Could you check a few things on this model? Use its own coordinates, in mm. A direction names the side the tool comes from. Coordinates: 2 decimals unless noted, no trailing zeros. Order: outer loops, then holes, each group sorted by start corner. A loop starts at its lowest first (then second) coordinate and runs counter-clockwise, first axis right, second up. Notation, with made-up numbers: (57.5, 33) - (101.5, 33) arc R33 ccw to (101.5, 67) - close; hole circle Ø6 at (33, 28.5). An arc over 180 degrees is marked (long way). One line per item, written item: value.
from build123d import *

# Parameters (mm, degrees)
F1_DEPTH = 500
F2_R     = 5
F3_DEPTH = 3.7
F4_R     = 5
F5_DEPTH = 41.001


with BuildPart() as f1:
    # F0 (on Top) → F1 (new body)
    with BuildSketch(Plane.XY):
        Polygon((0, 41), (0, 0), (41, 0), (41, 41), (31.4, 41), (31.4, 34), (34.8, 34), (34.8, 37.5), (37.3, 37.5), (37.3, 3.7), (3.7, 3.7), (3.7, 37.5), (6.2, 37.5), (6.2, 34), (9.6, 34), (9.6, 41), align=None)
    extrude(amount=F1_DEPTH)

    # F2 (on face) → F3 (cut, through all)
    with BuildSketch(Plane(origin=(0, 3.7, 0), x_dir=(-1, 0, 0), z_dir=(0, 1, 0))):
        with Locations((-20.5, 479.5)):
            Circle(F2_R)
        with Locations((-20.5, 20.5)):
            Circle(F2_R)
    extrude(amount=-F3_DEPTH, mode=Mode.SUBTRACT)

    # F4 (on face) → F5 (cut, through all)
    with BuildSketch(Plane(origin=(0, 0, 0), x_dir=(0, -1, 0), z_dir=(-1, 0, 0))):
        with Locations((-26, 20)):
            Circle(F4_R)
        with Locations((-26, 480)):
            Circle(F4_R)
    extrude(amount=-F5_DEPTH, mode=Mode.SUBTRACT)


solid = f1.part
Item 1: I want a section at D-D on z = 231.5. Please give me the cut outline in (x, y).
Conclusion:
outline: (0, 0) - (41, 0) - (41, 41) - (31.4, 41) - (31.4, 34) - (34.8, 34) - (34.8, 37.5) - (37.3, 37.5) - (37.3, 3.7) - (3.7, 3.7) - (3.7, 37.5) - (6.2, 37.5) - (6.2, 34) - (9.6, 34) - (9.6, 41) - (0, 41) - close
Item 2: I want a section at A-A on y = 26. Please give me the cut outline in (x, z), then the cut area to 3 significant figures.
Conclusion:
outline: (0, 0) - (3.7, 0) - (3.7, 15) - (0, 15) - close; (0, 25) - (3.7, 25) - (3.7, 475) - (0, 475) - close; (0, 485) - (3.7, 485) - (3.7, 500) - (0, 500) - close; (37.3, 0) - (41, 0) - (41, 15) - (37.3, 15) - close; (37.3, 25) - (41, 25) - (41, 475) - (37.3, 475) - close; (37.3, 485) - (41, 485) - (41, 500) - (37.3, 500) - close
area: 3,550 mm²
Item 3: For faces 4 (the face through (21.151, 1.876, 484.457)), 5 (the face through (21, 3.7, 246)), which set-ups out of +Z, -Z, +X, -X, +Y, -Y let a thin tool reach every point of the face, with its end or its side?
Conclusion:
face 4: +Y, -Y
face 5: +Z, -Z
Item 4: I want a section at B-B on y = 8. Please give me the cut outline in (x, z), then the cut area to 3 significant figures.
Conclusion:
outline: (0, 0) - (3.7, 0) - (3.7, 500) - (0, 500) - close; (37.3, 0) - (41, 0) - (41, 500) - (37.3, 500) - close
area: 3,700 mm²
Item 5: Thinking about a two-plate mould opening in Y: for faces 1 (the face through (36, 41, 246)), 2 (the face through (0, 21, 246)), 3 (the face through (39.124, 26.651, 484.957)), which applies, pulls with the +Y half, pulls with the -Y half, needs draft (parallel to the pull), parting line crosses it, or undercut?
Conclusion:
face 1: pulls with the +Y half
face 2: needs draft
face 3: undercut
Item 6: I want a section at C-C on x = 20.5. Please give me the cut outline in (y, z).
Conclusion:
outline: (0, 0) - (3.7, 0) - (3.7, 15.5) - (0, 15.5) - close; (0, 25.5) - (3.7, 25.5) - (3.7, 474.5) - (0, 474.5) - close; (0, 484.5) - (3.7, 484.5) - (3.7, 500) - (0, 500) - close
Item 7: If I drill on probe 1 along Z at (x, y) = (1, 26); probe 2 along X at (y, z) = (34.5, 425); probe 3 along X at (y, z) = (28, 433.5), over which ranges is the centre line in solid material (lowest first)?
Conclusion:
probe 1: 0 to 15, 25 to 475, 485 to 500
probe 2: 0 to 3.7, 6.2 to 9.6, 31.4 to 34.8, 37.3 to 41
probe 3: 0 to 3.7, 37.3 to 41
Item 8: I'm going to push a flat-ended pin straight in: pin 1 Ø9 at (y, z) = (26, 20) entering from -X. Where does the tip first touch, or does it pass through?
Conclusion:
pin 1: through
